Model file for the job. Use its own axes, mm. Round coordinates to 2 decimals unless told otherwise and drop trailing zeros. Loops run counter-clockwise (first coordinate to the right, second up) from the corner with the lowest first, then second, coordinate; pieces in that order, holes last. Notation, with made-up numbers: (0.5, 29.25) - (17.5, 29.25) arc R18 ccw to (17.5, 38.25) - close; hole circle Ø3 at (25, 39.25). An arc over 180 degrees is marked (long way). Use one line per item in the form item = value.
from build123d import *

# Parameters (mm, degrees)
F0_W      = 203.2
F0_H      = 9.271
F1_DEPTH  = 6.35
F2_W      = 127
F2_H      = 3.937
F3_DEPTH  = 3.683
F4_R      = 7.9375
F5_DEPTH  = 6.35
F6_R      = 5.08
F7_R      = 3.1115
F8_DEPTH  = 6.351
F9_W      = 9.525
F9_H      = 3.175
F10_DEPTH = 6.35


with BuildPart() as f1:
    # F0 (on Top) → F1 (new body)
    with BuildSketch(Plane.XY):
        with Locations((101.6, 4.6355)):
            Rectangle(F0_W, F0_H)
    extrude(amount=F1_DEPTH)

    # F2 (on face) → F3 (cut)
    with BuildSketch(Plane.XY.offset(6.35)):
        with Locations((139.7, 4.6355)):
            Rectangle(F2_W, F2_H)
    extrude(amount=-F3_DEPTH, mode=Mode.SUBTRACT)

    # F4 (on face) → F5 (join, through all)
    with BuildSketch(Plane.XY.offset(6.35)):
        with Locations((0, 4.6355)):
            Circle(F4_R)
    extrude(amount=-F5_DEPTH)

    # F6
    f6_edges = [f1.edges().sort_by_distance(p)[0] for p in [
        (6.443295, 9.271, 3.175),
        (6.443295, 0, 3.175),
    ]]
    fillet(f6_edges, radius=F6_R)

    # F7 (on face) → F8 (cut, through all)
    with BuildSketch(Plane.XY.offset(6.35)):
        with Locations((0, 4.6355)):
            Circle(F7_R)
    extrude(amount=-F8_DEPTH, mode=Mode.SUBTRACT)

    # F9 (on face) → F10 (join, through all)
    with BuildSketch(Plane.XY.offset(6.35)):
        with Locations((0.377471, 8.5725)):
            Rectangle(F9_W, F9_H)
    extrude(amount=-F10_DEPTH)


solid = f1.part
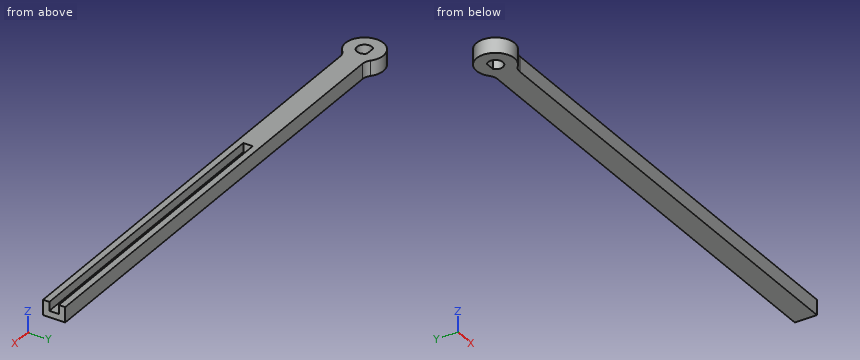
1. Flat gauge pins, fed straight in: pin 1 (1.1 mm diameter, centred on x = 123.5, z = 5, fed in from +Y); pin 2 (1.9 mm diameter, centred on x = 120.5, z = 4.5, fed in from -Y); pin 3 (3 mm diameter, centred on x = 124, y = 4.5, fed in from +Z). Where does each tip first touch, or does it go through?
Geometry check:
pin_1 = 9.27
pin_2 = 0
pin_3 = 2.67
2. Cut at A-A, the plane x = 0. Give the cut face in (y, z) (3 decimals).
Geometry check:
outline = (-3.302, 0) - (1.524, 0) - (1.524, 6.35) - (-3.302, 6.35) - close; (6.985, 0) - (12.573, 0) - (12.573, 6.35) - (6.985, 6.35) - close
3. Cut at B-B, the plane z = 1. Give the cut face in (x, y) (1 decimal).
Geometry check:
outline = (5.3, -1.3) arc R5.1 cw to (8.7, 0) - (203.2, 0) - (203.2, 9.3) - (8.7, 9.3) arc R5.1 cw to (5.3, 10.6) arc R7.9 ccw (long way) to start; hole (-2, 7) arc R3.1 ccw (long way) to (2, 7) - close
4. Cut at C-C, the plane x = 137. Give the cut face in (y, z), plus the area to 3 significant figures.
Geometry check:
outline = (0, 0) - (9.27, 0) - (9.27, 6.35) - (6.6, 6.35) - (6.6, 2.67) - (2.67, 2.67) - (2.67, 6.35) - (0, 6.35) - close
area = 44.4 mm^2
5. Wall check: probe 1 along Y at (x, z) = (139, 2.75); probe 2 along Z at (x, y) = (108.5, 4.5); probe 3 along Y at (x, z) = (162.5, 1.5). Give the ranges that are in metal, low to high.
Geometry check:
probe_1 = 0 to 2.67, 6.6 to 9.27
probe_2 = 0 to 2.67
probe_3 = 0 to 9.27
